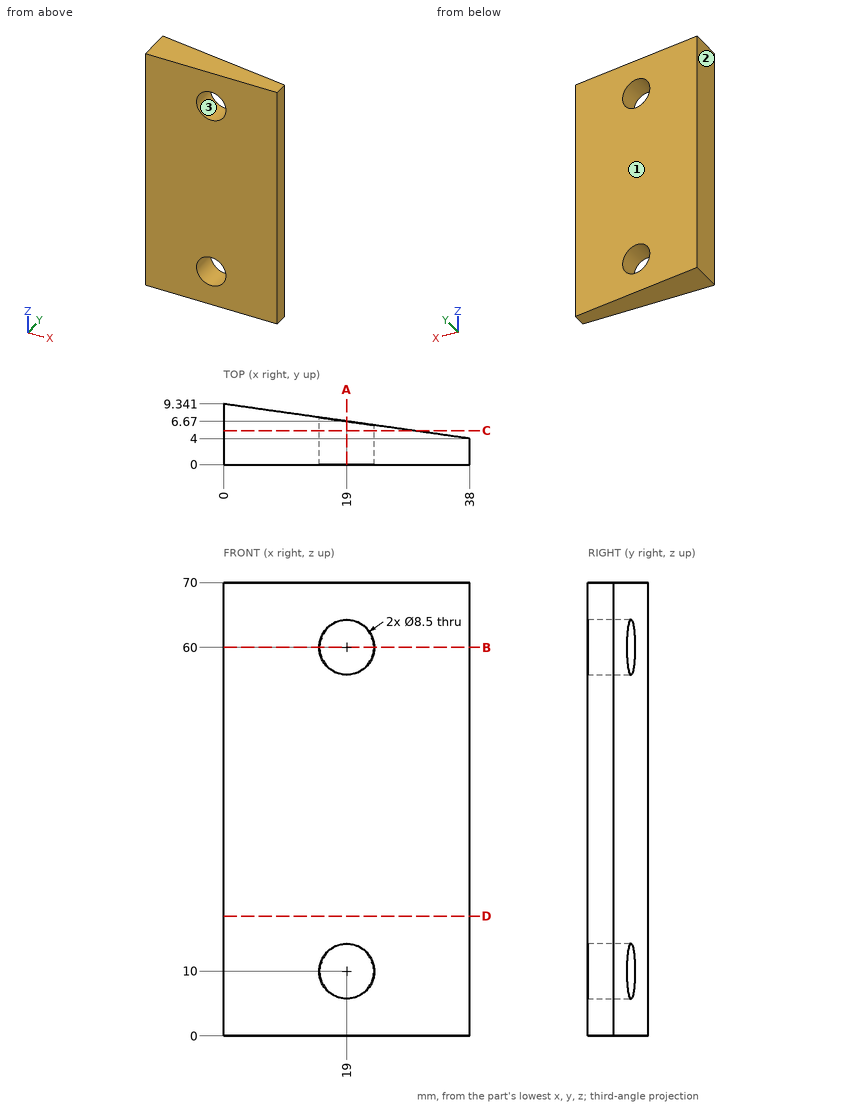
The figure shows three views and two pictorial views of one solid part (mm, origin at its lowest corner). Answer the questions. Round coordinates to 2 decimals unless told otherwise and drop trailing zeros. Write each loop counter-clockwise with the first axis right and the second up, starting at its lowest first coordinate (ties: lowest second). Pieces come first, ordered by that corner, then holes. Notation, with made-up numbers: (74.5, 87.5) - (106.5, 87.5) arc R19 ccw to (106.5, 114.5) - close; hole circle Ø8 at (89.25, 49). An arc over 180 degrees is marked (long way). Use one line per item in the form item = value. Start each with the question number.
Item 1: Determine the mould class of the marked faces 1, 2 and 3 for opening direction X: +X half, -X half, draft (parallel to the pull), parting line (faces both ways), or undercut.
Item 2: A cutting plane is placed at B-B (z = 60). Write down the section's boundary in (x, y), plus the area to 3 significant figures.
Item 3: A cutting plane is placed at C-C (y = 5.25). Give the number of separate pieces and of enclosed holes in the cut face, plus the area to 3 significant figures.
Item 4: Find the intervals of material crossed by line 1 (Z direction, x = 19, y = 5.5); line 2 (X direction, y = 2.5, z = 60); line 3 (X direction, y = 3.25, z = 63), in increasing order. Write a range as [from, to].
Item 5: A cutting plane is placed at D-D (z = 18.5). Write down the section's boundary in (x, y).
Item 6: Flat-ended cylindrical pins translate along their axes: pin 1 Ø3 at (x, z) = (6.5, 16.5) entering from +Y; pin 2 Ø12 at (x, z) = (31, 48.5) entering from +Y; pin 3 Ø7.5 at (x, z) = (19, 10) entering from +Y; pin 4 Ø1.5 at (x, z) = (13.5, 37.5) entering from +Y. Find the tip coordinate at first contact, or state that the pin passes through.
Item 7: A cutting plane is placed at A-A (x = 19). Write down the section's boundary in (y, z).
The answers:
q1.face_1 = +X half
q1.face_2 = -X half
q1.face_3 = undercut
q2.outline = (0, 0) - (14.75, 0) - (14.75, 7.27) - (0, 9.34) - close; (23.25, 0) - (38, 0) - (38, 4) - (23.25, 6.07) - close
q2.area = 197 mm^2
q3.separate_pieces = 1
q3.enclosed_holes = 2
q3.area = 1,920 mm^2
q4.line_1 = [0, 5.75], [14.25, 55.75], [64.25, 70]
q4.line_2 = [0, 14.75], [23.25, 38]
q4.line_3 = [0, 15.99], [22.01, 38]
q5.outline = (0, 0) - (38, 0) - (38, 4) - (0, 9.34) - close
q6.pin_1 = 8.64
q6.pin_2 = 5.83
q6.pin_3 = through
q6.pin_4 = 7.55
q7.outline = (0, 0) - (6.67, 0) - (6.67, 5.75) - (0, 5.75) - close; (0, 14.25) - (6.67, 14.25) - (6.67, 55.75) - (0, 55.75) - close; (0, 64.25) - (6.67, 64.25) - (6.67, 70) - (0, 70) - close
